Input: part model. Units: mm. Frame: model coordinates. Give positions to 0.01 mm unless a question says otherwise; leave off trailing zeros. Write each loop counter-clockwise with the first axis right and the second up, starting at its lowest first coordinate (ties: lowest second). Pieces come first, ordered by that corner, then holes. Notation, with made-up numbers: (-36.75, -30.75) - (5.25, -30.75) arc R23 cw to (5.25, -1.75) - close; hole circle Ø8 at (31.25, 78). An arc over 180 degrees is marked (long way). Answer as a JSON object with one key per item and string values. Group by question number.
from build123d import *

# Parameters (mm, degrees)
SKETCH1_R                = 32.5
SKETCH1_R_2              = 21
BOSS_EXTRUDE2_DEPTH      = 3
SKETCH2_R                = 1.75
CUT_EXTRUDE2_DEPTH       = 1
CUT_EXTRUDE2_DEPTH_BACK  = 4
SKETCH5_R                = 1.75
CUT_EXTRUDE4_DEPTH       = 1
CUT_EXTRUDE4_DEPTH_BACK  = 4
SKETCH13_R               = 1.75
CUT_EXTRUDE12_DEPTH      = 1
CUT_EXTRUDE12_DEPTH_BACK = 4


with BuildPart() as part:
    # Sketch1 → Boss-Extrude2 (new body)
    with BuildSketch(Plane(origin=(0, 0, 0), x_dir=(1, 0, 0), z_dir=(0, 1, 0))):
        Circle(SKETCH1_R)
        Circle(SKETCH1_R_2, mode=Mode.SUBTRACT)
    extrude(amount=BOSS_EXTRUDE2_DEPTH)

    # Sketch2 → Cut-Extrude2 (cut, two sides)
    with BuildSketch(Plane(origin=(0, 3, 0), x_dir=(1, 0, 0), z_dir=(0, 1, 0))) as cut_extrude2_sk:
        with Locations((0, -27.788884535)):
            Circle(SKETCH2_R)
    extrude(amount=CUT_EXTRUDE2_DEPTH, mode=Mode.SUBTRACT)
    extrude(cut_extrude2_sk.sketch, amount=-CUT_EXTRUDE2_DEPTH_BACK, mode=Mode.SUBTRACT)

    # Sketch5 → Cut-Extrude4 (cut, two sides)
    with BuildSketch(Plane(origin=(0, 3, 0), x_dir=(1, 0, 0), z_dir=(0, 1, 0))) as cut_extrude4_sk:
        with Locations((0.057759675, 27.766269398)):
            Circle(SKETCH5_R)
    extrude(amount=CUT_EXTRUDE4_DEPTH, mode=Mode.SUBTRACT)
    extrude(cut_extrude4_sk.sketch, amount=-CUT_EXTRUDE4_DEPTH_BACK, mode=Mode.SUBTRACT)

    # Sketch13 → Cut-Extrude12 (cut, two sides)
    with BuildSketch(Plane(origin=(0, 3, 0), x_dir=(1, 0, 0), z_dir=(0, 1, 0))) as cut_extrude12_sk:
        with Locations((-28.027387252, -0.003979104)):
            Circle(SKETCH13_R)
        with Locations((28.01619309, 0)):
            Circle(SKETCH13_R)
    extrude(amount=CUT_EXTRUDE12_DEPTH, mode=Mode.SUBTRACT)
    extrude(cut_extrude12_sk.sketch, amount=-CUT_EXTRUDE12_DEPTH_BACK, mode=Mode.SUBTRACT)


solid = part.part
1) Pin query (flat end, axial travel): P1, Ø12, axis at x = 4, z = -10, coming from the +Y side; P2, Ø4.5, axis at x = 0, z = 27.79, coming from the -Y side. Return the tip coordinate at first contact, or that it passes through.
2) Cut plane C-C on x = 0. Return the cut outline in (y, z).
3) Cut plane A-A on z = 5.5. Return the cut outline in (x, y), and give its area (3 significant figures).
4) Mould query, pull axis Z, two halves, no side actions, for faces 1 (the face through (0.81, 1.52, 29.34)), 2 (the face through (21.2, 0, -0.5)), 3 (the face through (31, 1.48, -9.76)). Classes: +Z half, -Z half, draft (parallel to the pull), parting line (faces both ways), or undercut.
5) Line query: line 1 along X through (y, z) = (0.6, 0); line 2 along Z through (x, y) = (0, 1); line 3 along Z through (x, y) = (-17.5, 2.6). Output: solid intervals per line, ascending. Write a range as from..to.
6) Cut plane B-B on x = 18. Return the cut outline in (y, z).
7) Cut plane D-D on y = 1.9. Return the cut outline in (x, z).
Filled in:
{
 "1": {"P1": "passes through", "P2": "stops at y = 0"},
 "2": {"outline": "(0, -32.5) - (3, -32.5) - (3, -29.52) - (0, -29.52) - close; (0, -26.02) - (3, -26.02) - (3, -21) - (0, -21) - close; (0, 21) - (3, 21) - (3, 26.04) - (0, 26.04) - close; (0, 29.54) - (3, 29.54) - (3, 32.5) - (0, 32.5) - close"},
 "3": {"outline": "(-32.03, 0) - (-20.27, 0) - (-20.27, 3) - (-32.03, 3) - close; (20.27, 0) - (32.03, 0) - (32.03, 3) - (20.27, 3) - close", "area": "70.6 mm²"},
 "4": {"face 1": "undercut", "face 2": "draft", "face 3": "parting line"},
 "5": {"line 1": "x = -32.5..-29.78, -26.28..-21, 21..26.27, 29.77..32.5", "line 2": "z = -32.5..-29.52, -26.02..-21, 21..26.04, 29.54..32.5", "line 3": "z = -27.39..-11.61, 11.61..27.39"},
 "6": {"outline": "(0, -27.06) - (3, -27.06) - (3, -10.82) - (0, -10.82) - close; (0, 10.82) - (3, 10.82) - (3, 27.06) - (0, 27.06) - close"},
 "7": {"outline": "circle Ø65 at (0, 0); hole circle Ø3.5 at (-28.03, 0); hole circle Ø42 at (0, 0); hole circle Ø3.5 at (0, 27.79); hole circle Ø3.5 at (0.06, -27.77); hole circle Ø3.5 at (28.02, 0)"}
}
